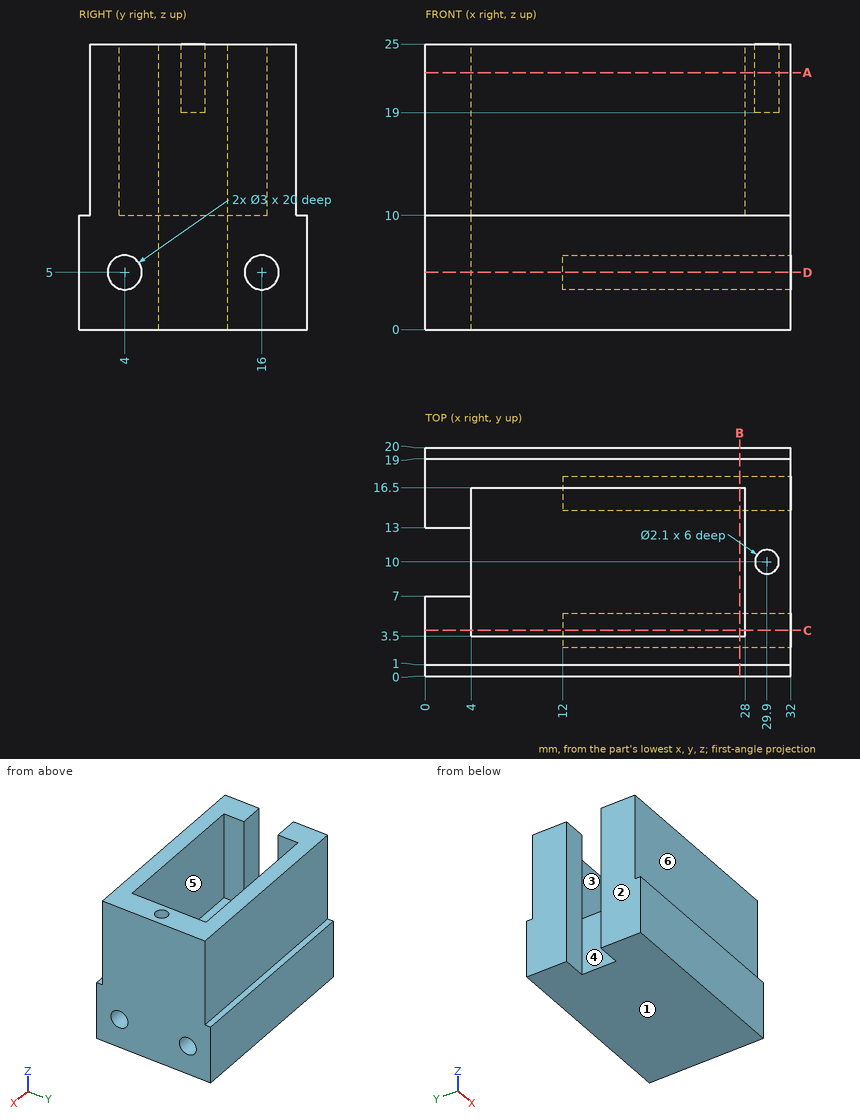
Could you check a few things on this drawing? It's one solid part, dimensions in mm from its lowest x, y, z. A direction names the side the tool comes from. Round coordinates to 2 decimals unless told otherwise and drop trailing zeros. Order: outer loops, then holes, each group sorted by start corner. A loop starts at its lowest first (then second) coordinate and runs counter-clockwise, first axis right, second up. Notation, with made-up numbers: (-2, 37.5) -> (30, 37.5) arc R13 cw to (30, 60.5) -> close; hole circle Ø5 at (59.5, 76). An arc over 180 degrees is marked (long way). One line per question, with ' | ' between items.
Q1. I'm going to push flat-ended pins straight in: pin 1 (3 mm diameter, centred on y = 9.5, z = 6.5, fed in from -X); pin 2 (0.6 mm diameter, centred on x = 30, y = 10, fed in from +Z); pin 3 (1.2 mm diameter, centred on x = 3, z = 13, fed in from -Y). Where does each tip first touch, or does it pass through?
Computed values:
pin 1: x = 4 | pin 2: z = 19 | pin 3: y = 1
Q2. If we section it at B-B on x = 27.5: Write out the boundary of the cut face in (y, z), plus the area to 3 significant figures.
Computed values:
outline: (0, 0) -> (20, 0) -> (20, 10) -> (19, 10) -> (19, 25) -> (16.5, 25) -> (16.5, 10) -> (3.5, 10) -> (3.5, 25) -> (1, 25) -> (1, 10) -> (0, 10) -> close; hole circle Ø3 at (4, 5); hole circle Ø3 at (16, 5) | area: 261 mm²
Q3. If we section it at C-C on y = 4: Write out the boundary of the cut face in (x, z).
Computed values:
outline: (0, 0) -> (32, 0) -> (32, 3.5) -> (12, 3.5) -> (12, 6.5) -> (32, 6.5) -> (32, 25) -> (28, 25) -> (28, 10) -> (4, 10) -> (4, 25) -> (0, 25) -> close
Q4. If we section it at A-A on z = 22.5: Write out the boundary of the cut face in (x, y).
Computed values:
outline: (0, 1) -> (32, 1) -> (32, 19) -> (0, 19) -> (0, 13) -> (4, 13) -> (4, 16.5) -> (28, 16.5) -> (28, 3.5) -> (4, 3.5) -> (4, 7) -> (0, 7) -> close; hole circle Ø2.1 at (29.9, 10)
Q5. If I drill on line 1 (Y direction, x = 16, z = 12); line 2 (X direction, y = 14.25, z = 17); line 3 (Y direction, x = 29.9, z = 22.25), over which ranges is the centre line in solid material (lowest first)? Write a range as from..to.
Computed values:
line 1: 1..3.5, 16.5..19 | line 2: 0..4, 28..32 | line 3: 1..8.95, 11.05..19
Q6. We'd pull the mould along X, two halves only. Please class the marked faces 1, 2 and 3: released by +X, released by -X, zero draft, split by the parting line, or undercut.
Computed values:
face 1: zero draft | face 2: released by -X | face 3: undercut
Q7. Which directions (+Z, -Z, +X, -X, +Y, -Y) give clear straight access to the entire face, cutting with the end or side of a thin tool? Please do the marked faces 4, 5 and 6.
Computed values:
face 4: +Z, -Z, -X | face 5: +Z | face 6: +Z, +X, -X, -Y
Q8. If we section it at D-D on z = 5: Write out the boundary of the cut face in (x, y).
Computed values:
outline: (0, 0) -> (32, 0) -> (32, 2.5) -> (12, 2.5) -> (12, 5.5) -> (32, 5.5) -> (32, 14.5) -> (12, 14.5) -> (12, 17.5) -> (32, 17.5) -> (32, 20) -> (0, 20) -> (0, 13) -> (4, 13) -> (4, 7) -> (0, 7) -> close
